Work out the finished part from the listing and answer in its coordinate system (mm). A direction names the side the tool comes from. Coordinates: 2 decimals unless noted, no trailing zeros. Order: outer loops, then holes, each group sorted by start corner. A loop starts at its lowest first (then second) coordinate and runs counter-clockwise, first axis right, second up. Notation, with made-up numbers: M 10.5,55 L 28.5,55 A36 cw 28.5,91 Z; hole C 32,58.5 d9. An arc over 180 degrees is marked long. Use a Markdown table: item, result. Add a question column.
Autodesk Inventor part; units mm, degrees
ref_plane "YZ Plane" through (0, 0, 0) normal (1, 0, 0) x (0, 1, 0)
ref_plane "XZ Plane" through (0, 0, 0) normal (0, 1, 0) x (-1, 0, 0)
ref_plane "XY Plane" through (0, 0, 0) normal (0, 0, 1) x (1, 0, 0)
sketch "Sketch1" plane through (0, 0, 0) normal (0, 1, 0) x (-1, 0, 0)
  line L0 (66.6667, 111.1111) -> (-183.3333, 111.1111)
  line L1 (-183.3333, 111.1111) -> (-183.3333, -88.8889)
  line L2 (-183.3333, -88.8889) -> (66.6667, -88.8889)
  line L3 (66.6667, -88.8889) -> (66.6667, 111.1111)
  point P0 (0, 0)
  dimension "d0" = 200
  dimension "d1" = 250
extrude "Extrusion1" add sketch "Sketch1" along normal blind 12
sketch "Sketch2" plane through (0, 12, 0) normal (0, 1, 0) x (1, 0, 0)
  line L0 (183.3333, -111.1111) -> (183.3333, 88.8889)
  line L1 (183.3333, 88.8889) -> (-66.6667, 88.8889)
  line L2 (-66.6667, 88.8889) -> (-66.6667, -111.1111)
  line L3 (-66.6667, -111.1111) -> (183.3333, -111.1111)
  line L4 (-46.6667, -91.1111) -> (-46.6667, 68.8889)
  line L5 (-46.6667, 68.8889) -> (163.3333, 68.8889)
  line L6 (163.3333, 68.8889) -> (163.3333, -91.1111)
  line L7 (163.3333, -91.1111) -> (-46.6667, -91.1111)
  line L8 (-46.6667, -91.1111) -> (163.3333, 68.8889)
  line L9 (163.3333, -91.1111) -> (-46.6667, 68.8889)
  line L10 (160.9092, -94.2928) -> (-49.0908, 65.7072)
  line L11 (165.7575, -87.9294) -> (-44.2425, 72.0706)
  line L12 (-49.0908, -87.9294) -> (160.9092, 72.0706)
  line L13 (-44.2425, -94.2928) -> (165.7575, 65.7072)
  point P0 (0, 0)
  point P1 (58.3333, -16.1398)
  point P2 (-40.0665, -91.1111)
  point P3 (156.7331, -91.1111)
  point P4 (163.3333, 63.8602)
  point P5 (64.9335, -11.1111)
  point P6 (163.3333, -86.0824)
  point P7 (58.3333, -6.0824)
  point P8 (156.7331, 68.8889)
  point P9 (-40.0665, 68.8889)
  point P10 (-46.6667, -86.0824)
  point P11 (51.7331, -11.1111)
  point P12 (-46.6667, 63.8602)
  dimension "d4" = 20
  dimension "d5" = 4
  dimension "d6" = 4
  dimension "d7" = 4
  dimension "d8" = 4
extrude "Extrusion2" cut sketch "Sketch2" against normal blind 6 contours L4 L10 L12 | L13 L10 L7 | L5 L12 L11 | L11 L13 L6
properties part number "planeDerzavki" material "Aluminum 6061"
(1) The mould has two halves that part along Z. Classify faces 1 (the flat face through (57, 6, 111.111)), 2 (the flat face through (-66.667, 6, 10)), 3 (the flat face through (108.22, 9.04, 54.15)): pulls with the +Z half, pulls with the -Z half, needs draft (parallel to the pull), parting line crosses it, or undercut.
(2) Which of the six approach directions +Z, -Z, +X, -X, +Y, -Y give full straight-line access (tool end or side, diameter ignored) to faces 4 (the flat face through (60, 9, 91.111)), 5 (the flat face through (183.333, 6, 13))?
(3) A cutting plane is placed at C-C on z = -60.5. Write down the section's boundary in (x, y), plus the area to 3 significant figures.
(4) Straight lines are drawn through the part: line 1 (X direction, y = 10, z = 17.5); line 2 (X direction, y = 10.5, z = 13.5); line 3 (Z direction, x = -6, y = 11.25). For each, find the intervals that lie inside material, in ascending order.
(5) Given P1, Ø6, axis at x = 107, z = 29.5, coming from the +Y side, flat-ended and moving along its own axis, determine where the tip first touches the part or whether it passes through.
(6) A cutting plane is placed at B-B on x = 88. Write down the section's boundary in (y, z).
(7) A cutting plane is placed at A-A on y = 9.5. Write down the section's boundary in (x, z), plus the area to 3 significant figures.
From the geometry:
| question | item | result |
|---|---|---|
| 1 | face 1 | pulls with the +Z half |
| 1 | face 2 | needs draft |
| 1 | face 3 | undercut |
| 2 | face 4 | +Y |
| 2 | face 5 | +Z, -Z, +X, +Y, -Y |
| 3 | outline | M -66.67,0 L 183.33,0 L 183.33,12 L 163.33,12 L 163.33,6 L 158.92,6 L 158.92,12 L 145.72,12 L 145.72,6 L -29.06,6 L -29.06,12 L -42.26,12 L -42.26,6 L -46.67,6 L -46.67,12 L -66.67,12 Z |
| 3 | area | 1,900 mm2 |
| 4 | line 1 | x = -66.67 to -46.67, 43.35 to 56.55, 60.12 to 73.32, 163.33 to 183.33 |
| 4 | line 2 | x = -66.67 to -46.67, 48.6 to 68.07, 163.33 to 183.33 |
| 4 | line 3 | z = -88.89 to -68.89, -42.93 to -32.88, 55.1 to 65.16, 91.11 to 111.11 |
| 5 | P1 | stops at y = 6 |
| 6 | outline | M 0,-88.89 L 12,-88.89 L 12,-68.89 L 6,-68.89 L 6,-16.52 L 12,-16.52 L 12,-6.46 L 6,-6.46 L 6,28.69 L 12,28.69 L 12,38.74 L 6,38.74 L 6,91.11 L 12,91.11 L 12,111.11 L 0,111.11 Z |
| 7 | outline | M -66.67,-88.89 L 183.33,-88.89 L 183.33,111.11 L -66.67,111.11 Z; hole M -46.67,-63.86 L 51.73,11.11 L -46.67,86.08 Z; hole M -40.07,-68.89 L 156.73,-68.89 L 58.33,6.08 Z; hole M -40.07,91.11 L 58.33,16.14 L 156.73,91.11 Z; hole M 64.93,11.11 L 163.33,-63.86 L 163.33,86.08 Z |
| 7 | area | 20,500 mm2 |
